```python
from build123d import *

# Parameters (mm, degrees)
F0_R     = 12.7
F1_DEPTH = 44.45
F2_DEPTH = 12.7


with BuildPart() as f1:
    # F0 (on Front) → F1 (new body)
    with BuildSketch(Plane.XZ):
        with BuildLine():
            Line((-31.75, 0), (0, 0))
            Line((0, 0), (31.75, 0))
            Line((31.75, 0), (31.75, 8.89))
            Line((31.75, 8.89), (12.7, 8.89))
            Line((12.7, 8.89), (12.7, 21.59))
            Line((12.7, 21.59), (63.5, 21.59))
            Line((63.5, 21.59), (63.5, 34.29))
            Line((63.5, 34.29), (47.625, 34.29))
            Line((47.625, 34.29), (21.0935941582, 73.8409400841))
            ThreePointArc((21.0935941582, 73.8409400841), (12.0532981257, 82.0489700372), (0.2274431955, 85.09))
            Line((0.2274431955, 85.09), (-0.2274431955, 85.09))
            ThreePointArc((-0.2274431955, 85.09), (-12.0532981257, 82.0489700372), (-21.0935941582, 73.8409400841))
            Line((-21.0935941582, 73.8409400841), (-47.625, 34.29))
            Line((-47.625, 34.29), (-63.5, 34.29))
            Line((-63.5, 34.29), (-63.5, 21.59))
            Line((-63.5, 21.59), (-12.7, 21.59))
            Line((-12.7, 21.59), (-12.7, 8.89))
            Line((-12.7, 8.89), (-31.75, 8.89))
            Line((-31.75, 8.89), (-31.75, 0))
        make_face()
        with Locations((0, 59.6910183355)):
            Circle(F0_R, mode=Mode.SUBTRACT)
    extrude(amount=F1_DEPTH)

    # F0 (on Front) → F2 (join)
    with BuildSketch(Plane.XZ):
        with BuildLine():
            Line((-31.75, 0), (0, 0))
            Line((0, 0), (31.75, 0))
            Line((31.75, 0), (31.75, 8.89))
            Line((31.75, 8.89), (12.7, 8.89))
            Line((12.7, 8.89), (12.7, 21.59))
            Line((12.7, 21.59), (63.5, 21.59))
            Line((63.5, 21.59), (63.5, 34.29))
            Line((63.5, 34.29), (47.625, 34.29))
            Line((47.625, 34.29), (21.0935941582, 73.8409400841))
            ThreePointArc((21.0935941582, 73.8409400841), (12.0532981257, 82.0489700372), (0.2274431955, 85.09))
            Line((0.2274431955, 85.09), (-0.2274431955, 85.09))
            ThreePointArc((-0.2274431955, 85.09), (-12.0532981257, 82.0489700372), (-21.0935941582, 73.8409400841))
            Line((-21.0935941582, 73.8409400841), (-47.625, 34.29))
            Line((-47.625, 34.29), (-63.5, 34.29))
            Line((-63.5, 34.29), (-63.5, 21.59))
            Line((-63.5, 21.59), (-12.7, 21.59))
            Line((-12.7, 21.59), (-12.7, 8.89))
            Line((-12.7, 8.89), (-31.75, 8.89))
            Line((-31.75, 8.89), (-31.75, 0))
        make_face()
        with Locations((0, 59.6910183355)):
            Circle(F0_R, mode=Mode.SUBTRACT)
        with BuildLine():
            Line((47.625, 34.29), (63.5, 34.29))
            Line((63.5, 34.29), (63.5, 85.09))
            Line((63.5, 85.09), (0.2274431955, 85.09))
            ThreePointArc((0.2274431955, 85.09), (12.0532981257, 82.0489700372), (21.0935941582, 73.8409400841))
            Line((21.0935941582, 73.8409400841), (47.625, 34.29))
        make_face()
        with BuildLine():
            Line((-63.5, 85.09), (-63.5, 34.29))
            Line((-63.5, 34.29), (-47.625, 34.29))
            Line((-47.625, 34.29), (-21.0935941582, 73.8409400841))
            ThreePointArc((-21.0935941582, 73.8409400841), (-12.0532981257, 82.0489700372), (-0.2274431955, 85.09))
            Line((-0.2274431955, 85.09), (-63.5, 85.09))
        make_face()
    extrude(amount=F2_DEPTH)


solid = f1.part
```
Could you check a few things on this model? Use its own coordinates, in mm. A direction names the side the tool comes from. Coordinates: 2 decimals unless noted, no trailing zeros. Write each loop counter-clockwise with the first axis right and the second up, starting at its lowest first coordinate (ties: lowest second). Pieces come first, ordered by that corner, then holes. Notation, with made-up numbers: M 67,-11.75 L 123,-11.75 A18 cw 123,-1.75 Z; hole C 89.5,85.25 d1. An arc over 180 degrees is marked long. Answer as CSV lines item,"result". Start each with the question number.
1) For faces 1 (the flat face through (31.75, -22, 4)), 2 (the flat face through (22, -22, 8.89)), 3 (the flat face through (-46, -12.7, 66)), 4 (the flat face through (45, -12.7, 66)), 5 (the flat face through (-38, -22, 21.59)), which set-ups out of +Z, -Z, +X, -X, +Y, -Y let a thin tool reach every point of the face, with its end or its side?
2) For P1, Ø10, axis at y = -24.5, z = 15.5, coming from the +X side; P2, Ø4.5, axis at y = -19, z = 2.5, coming from the -X side; P3, Ø5.5, axis at x = 23.5, y = -23.5, coming from the +Z side, each with a flat end and sliding along its axis, tell me the tip position at first contact or that it passes through.
3) I want a section at B-B, the plane x = 14. Please give me the cut outline in (y, z), and give its area (3 significant figures).
4) We'd pull the mould along Z, two halves only. Please class faces 6 (the flat face through (-55, -28, 34.29)), 7 (the flat face through (63.5, -12, 46)), 8 (the flat face through (12.7, -22, 15)): +Z half, -Z half, draft (parallel to the pull), parting line (faces both ways), or undercut.
5) Please list where these lines run through material, in increasing order: line 1 (Z direction, x = 0, y = -18); line 2 (Z direction, x = -50, y = -39.5); line 3 (Z direction, x = 31, y = -7). Write a range as from..to.
6) I want a section at C-C, the plane y = -3. Please give me the cut outline in (x, z), and give its area (3 significant figures).
7) I want a section at D-D, the plane x = -39.5. Please give me the cut outline in (y, z), and give its area (3 significant figures).
8) I want a section at A-A, the plane z = 57. Please give me the cut outline in (x, y).
Data:
1,face 1,"-Z, +X, +Y, -Y"
1,face 2,"+X, +Y, -Y"
1,face 3,"+Z, -X, -Y"
1,face 4,"+Z, +X, -Y"
1,face 5,"-X, +Y, -Y"
2,P1,"stops at x = 12.7"
2,P2,"stops at x = -31.75"
2,P3,"stops at z = 74.34"
3,outline,"M -44.45,0 L 0,0 L 0,8.89 L -44.45,8.89 Z; M -44.45,21.59 L 0,21.59 L 0,85.09 L -12.7,85.09 L -12.7,80.88 L -44.45,80.88 Z"
3,area,"3,080 mm^2"
4,face 6,"+Z half"
4,face 7,"draft"
4,face 8,"undercut"
5,line 1,"z = 0..46.99, 72.39..85.09"
5,line 2,"z = 21.59..34.29"
5,line 3,"z = 0..8.89, 21.59..85.09"
6,outline,"M -63.5,21.59 L -12.7,21.59 L -12.7,8.89 L -31.75,8.89 L -31.75,0 L 31.75,0 L 31.75,8.89 L 12.7,8.89 L 12.7,21.59 L 63.5,21.59 L 63.5,85.09 L -63.5,85.09 Z; hole C 0,59.69 d25.4"
6,area,"8,440 mm^2"
7,outline,"M -44.45,21.59 L 0,21.59 L 0,85.09 L -12.7,85.09 L -12.7,46.4 L -44.45,46.4 Z"
7,area,"1,590 mm^2"
8,outline,"M -63.5,-12.7 L -32.39,-12.7 L -32.39,-44.45 L -12.41,-44.45 L -12.41,0 L -63.5,0 Z; M 12.41,-44.45 L 32.39,-44.45 L 32.39,-12.7 L 63.5,-12.7 L 63.5,0 L 12.41,0 Z"
